The model under review builds one solid part; all positions refer to its coordinate system, in mm. A direction names the side the tool comes from. Coordinates: 2 decimals unless noted, no trailing zeros. Order: outer loops, then holes, each group sorted by start corner. A loop starts at its lowest first (then second) coordinate and runs counter-clockwise, first axis right, second up. Notation, with made-up numbers: (53.5, 64) -> (75.5, 64) arc R22 ccw to (75.5, 71) -> close; hole circle Ø2 at (-33.5, 53.25). An arc over 180 degrees is marked (long way). Use CSV: the item, a comma, the result in double quotes. Start each with the question number.
```python
from build123d import *

# Parameters (mm, degrees)
BOSS_EXTRUDE1_DEPTH      = 45.72
SHELL1_T                 = -2.54
SHELL1_THICKNESS_2_DEPTH = 7.62
SHELL1_THICKNESS_3_DEPTH = 7.62
BOSS_EXTRUDE2_DEPTH      = 5.08
SKETCH3_R                = 6.35
CUT_EXTRUDE1_DEPTH       = 45.72
SKETCH4_W                = 5.08
SKETCH4_H                = 2.54
BOSS_EXTRUDE3_DEPTH      = 5.08
SKETCH5_W                = 2.54
SKETCH5_H                = 5.08
BOSS_EXTRUDE4_DEPTH      = 2.54
SKETCH6_W                = 5.08
SKETCH6_H                = 1.27
BOSS_EXTRUDE5_DEPTH      = 1.27


with BuildPart() as part:
    # Sketch1 → Boss-Extrude1 (new body)
    with BuildSketch(Plane.XY):
        with BuildLine():
            Line((0, 0), (-19.05, -92.71))
            Line((-19.05, -92.71), (69.85, -92.71))
            Line((69.85, -92.71), (50.8, 0))
            ThreePointArc((50.8, 0), (25.4, 17.565060875), (0, 0))
        make_face()
    extrude(amount=BOSS_EXTRUDE1_DEPTH)

    # Shell1
    shell1_openings = [part.faces().sort_by_distance(p)[0] for p in [
        (25.4, -92.71, 22.86),
    ]]
    offset(amount=SHELL1_T, openings=shell1_openings, kind=Kind.INTERSECTION)

    # Shell1 thickness 2 face (on inner face of the shell) → Shell1 thickness 2 (add)
    with BuildSketch(Plane(origin=(25.4, -46.578295761, 43.18), x_dir=(1, 0, 0), z_dir=(0, 0, 1))):
        with BuildLine():
            Line((41.856932666, -46.131704239), (-41.856932666, -46.131704239))
            Line((-41.856932666, -46.131704239), (-22.953477125, 45.865112726))
            ThreePointArc((-22.953477125, 45.865112726), (0, 61.603356636), (22.953477125, 45.865112726))
            Line((22.953477125, 45.865112726), (41.856932666, -46.131704239))
        make_face()
    extrude(amount=-SHELL1_THICKNESS_2_DEPTH)

    # Shell1 thickness 3 face (on inner face of the shell) → Shell1 thickness 3 (add)
    with BuildSketch(Plane(origin=(25.4, -46.578295761, 2.54), x_dir=(-1, 0, 0), z_dir=(0, 0, -1))):
        with BuildLine():
            Line((41.856932666, -46.131704239), (-41.856932666, -46.131704239))
            Line((-41.856932666, -46.131704239), (-22.953477125, 45.865112726))
            ThreePointArc((-22.953477125, 45.865112726), (0, 61.603356636), (22.953477125, 45.865112726))
            Line((22.953477125, 45.865112726), (41.856932666, -46.131704239))
        make_face()
    extrude(amount=-SHELL1_THICKNESS_3_DEPTH)

    # Sketch2 → Boss-Extrude2 (add)
    with BuildSketch(Plane(origin=(0, 0, 35.56), x_dir=(-1, 0, 0), z_dir=(0, 0, -1))):
        with BuildLine():
            Line((-48.353477125, -0.713183035), (-67.256932666, -92.71))
            Line((-67.256932666, -92.71), (16.456932666, -92.71))
            Line((16.456932666, -92.71), (-2.446522875, -0.713183035))
            ThreePointArc((-2.446522875, -0.713183035), (-11.484590973, 10.712623327), (-25.4, 15.025060875))
            ThreePointArc((-25.4, 15.025060875), (-39.315409027, 10.712623327), (-48.353477125, -0.713183035))
        make_face()
    extrude(amount=BOSS_EXTRUDE2_DEPTH)

    # Sketch3 → Cut-Extrude1 (cut)
    with BuildSketch(Plane(origin=(0, 0, 0), x_dir=(-1, 0, 0), z_dir=(0, 0, -1))):
        with Locations((-25.4, -18.738085506)):
            Circle(SKETCH3_R)
    extrude(amount=-CUT_EXTRUDE1_DEPTH, mode=Mode.SUBTRACT)

    # Sketch4 → Boss-Extrude3 (add)
    with BuildSketch(Plane(origin=(2.488018693, -0.511236718, 0), x_dir=(0, 0, -1), z_dir=(0.979534919, -0.201274298, 0))):
        with Locations((-20.32, -45.602294641)):
            Rectangle(SKETCH4_W, SKETCH4_H)
    extrude(amount=BOSS_EXTRUDE3_DEPTH)

    # Sketch5 → Boss-Extrude4 (add)
    with BuildSketch(Plane(origin=(-8.922951498, -43.425030624, 0), x_dir=(0.979534919, -0.201274298, 0), z_dir=(0.201274298, 0.979534919, 0))):
        with Locations((6.35, -20.32)):
            Rectangle(SKETCH5_W, SKETCH5_H)
    extrude(amount=BOSS_EXTRUDE4_DEPTH)

    # Sketch6 → Boss-Extrude5 (add)
    with BuildSketch(Plane(origin=(4.976037387, -1.022473436, 0), x_dir=(0, 0, 1), z_dir=(-0.979534919, 0.201274298, 0))):
        with Locations((20.32, -42.427294641)):
            Rectangle(SKETCH6_W, SKETCH6_H)
    extrude(amount=BOSS_EXTRUDE5_DEPTH)


solid = part.part
```
Q1. Add section A-A, the plane x = 25.4. State the section outline as (y, z) points.
Q2. For faces 4 (the cylindrical face through (19.343, -16.831, 5.009)), 5 (the flat face through (-2.788, -42.093, 20.284)), 6 (the cylindrical face through (25.81, 15.02, 20.18)), list the 3-axis set-ups (+Z, -Z, +X, -X, +Y, -Y) from which the entire face can be reached by the end or side of a thin tool; tool diameter is ignored.
Q3. Clearance check with flat-ended pins moving along their axes: pin 1 Ø7.5 at (x, y) = (25.4, -18.74) entering from +Z; pin 2 Ø6 at (y, z) = (-33.5, 19) entering from -X. State where each tip first meets the part, or that it passes through.
Q4. Add section D-D, the plane x = 61.5. State the section outline as (y, z) points.
Q5. Add section C-C, the plane y = -84. State the section outline as (x, z) points.
Q6. Add section B-B, the plane z = 19.5. State the section outline as (x, y) points.
Q7. To check wall thickness, follow probe 1 along Y at (x, z) = (25.4, 34); probe 2 along Z at (x, y) = (43, -31.5); probe 3 along X at (y, z) = (2, 19). State the ranges of each line that lie inside material, in increasing order.
Q8. Draft analysis for pull direction Z (two halves, no side actions). For faces 1 (the flat face through (-9.392, -45.706, 22.54)), 2 (the flat face through (-1.466, -44.994, 20.356)), 3 (the flat face through (25, -49, 45.72)), state which applies: +Z half, -Z half, draft (parallel to the pull), parting line (faces both ways), or undercut.
Answer block:
1,outline,"(-92.71, 0) -> (-25.09, 0) -> (-25.09, 10.16) -> (-92.71, 10.16) -> close; (-92.71, 30.48) -> (-25.09, 30.48) -> (-25.09, 45.72) -> (-92.71, 45.72) -> close; (-12.39, 0) -> (17.57, 0) -> (17.57, 45.72) -> (-12.39, 45.72) -> (-12.39, 30.48) -> (15.03, 30.48) -> (15.03, 10.16) -> (-12.39, 10.16) -> close"
2,face 4,"+Z, -Z"
2,face 5,"none"
2,face 6,"-Y"
3,pin 1,"passes through"
3,pin 2,"stops at x = -7.5"
4,outline,"(-92.71, 0) -> (-52.07, 0) -> (-52.07, 45.72) -> (-92.71, 45.72) -> (-92.71, 30.48) -> (-64.69, 30.48) -> (-64.69, 10.16) -> (-92.71, 10.16) -> close"
5,outline,"(-17.26, 0) -> (68.06, 0) -> (68.06, 45.72) -> (-17.26, 45.72) -> close; hole (-14.67, 10.16) -> (65.47, 10.16) -> (65.47, 30.48) -> (-14.67, 30.48) -> close"
6,outline,"(-19.05, -92.71) -> (-16.46, -92.71) -> (-6.95, -46.42) -> (-1.97, -47.45) -> (-0.95, -42.47) -> (-4.68, -41.7) -> (-4.94, -42.95) -> (-3.69, -43.2) -> (-3.95, -44.45) -> (-6.43, -43.94) -> (2.45, -0.71) arc R24.61 cw to (48.35, -0.71) -> (67.26, -92.71) -> (69.85, -92.71) -> (50.8, 0) arc R27.15 ccw to (0, 0) -> close"
7,probe 1,"y = -92.71 to -25.09, -12.39 to 17.57"
7,probe 2,"z = 0 to 10.16, 30.48 to 45.72"
7,probe 3,"x = 0.85 to 3.69, 47.11 to 49.95"
8,face 1,"draft"
8,face 2,"undercut"
8,face 3,"+Z half"
